Autodesk Inventor part; units mm, degrees
ref_plane "YZ Plane" through (0, 0, 0) normal (1, 0, 0) x (0, 1, 0)
ref_plane "XZ Plane" through (0, 0, 0) normal (0, 1, 0) x (-1, 0, 0)
ref_plane "XY Plane" through (0, 0, 0) normal (0, 0, 1) x (1, 0, 0)
sketch "Sketch1" plane through (0, 0, 0) normal (0, 0, 1) x (1, 0, 0)
  line L0 (0, 0) -> (177.8, 0)
  line L1 (177.8, 0) -> (177.8, 101.6)
  line L2 (177.8, 101.6) -> (0, 101.6)
  line L3 (0, 101.6) -> (0, 0)
  arc A0 (25.4, 101.6) -> (0, 76.2) centre (25.4, 76.2) ccw
  arc A1 (177.8, 76.2) -> (152.4, 101.6) centre (152.4, 76.2) ccw
  arc A2 (152.4, 0) -> (177.8, 25.4) centre (152.4, 25.4) ccw
  arc A3 (0, 25.4) -> (25.4, 0) centre (25.4, 25.4) ccw
  arc A4 (88.9, 85.09) -> (54.61, 50.8) centre (88.9, 50.8) ccw construction
  arc A5 (88.9, 88.9) -> (50.8, 50.8) centre (88.9, 50.8) ccw
  arc A6 (88.9, 81.28) -> (58.42, 50.8) centre (88.9, 50.8) ccw
  arc A7 (88.9, 81.28) -> (88.9, 88.9) centre (88.9, 85.09) ccw
  arc A8 (50.8, 50.8) -> (58.42, 50.8) centre (54.61, 50.8) ccw
  line L4 (88.9, 50.8) -> (54.61, 50.8) construction
  line L5 (88.9, 50.8) -> (88.9, 85.09) construction
  arc A9 (88.9, 20.32) -> (119.38, 50.8) centre (88.9, 50.8) ccw
  line L6 (88.9, 50.8) -> (123.19, 50.8) construction
  arc A10 (88.9, 16.51) -> (123.19, 50.8) centre (88.9, 50.8) ccw construction
  arc A11 (127, 50.8) -> (119.38, 50.8) centre (123.19, 50.8) ccw
  arc A12 (88.9, 12.7) -> (127, 50.8) centre (88.9, 50.8) ccw
  arc A13 (88.9, 20.32) -> (88.9, 12.7) centre (88.9, 16.51) ccw
  line L7 (0, 50.8) -> (177.8, 50.8)
  line L8 (88.9, 101.6) -> (88.9, 0)
  circle A14 centre (12.7, 71.882) radius 6.35
  circle A15 centre (33.02, 71.882) radius 6.35
  circle A16 centre (12.7, 29.718) radius 6.35
  circle A17 centre (33.02, 29.718) radius 6.35
  circle A18 centre (165.1, 29.718) radius 6.35
  circle A19 centre (144.78, 29.718) radius 6.35
  circle A20 centre (165.1, 71.882) radius 6.35
  circle A21 centre (144.78, 71.882) radius 6.35
  point P0 (0, 0)
  point P1 (0, 0)
  point P2 (-19.4884, -65.4138)
  dimension "d2" = 177.8
  dimension "d3" = 101.6
  dimension "d4" = 50.8
  dimension "d5" = 50.8
  dimension "d6" = 50.8
  dimension "d7" = 50.8
  dimension "d9" = 50.8
  dimension "d10" = 88.9
  dimension "d11" = 34.29
  dimension "d12" = 90
  dimension "d13" = 7.62
  dimension "d14" = 360
  dimension "d15" = 0
  dimension "d16" = 0
  dimension "d17" = 0
  dimension "d19" = 0
  dimension "d20" = 12.7
  dimension "d21" = 12.7
  dimension "d22" = 20.32
  dimension "d24" = 21.082
  dimension "d25" = 12.7
extrude "Extrusion1" add sketch "Sketch1" along normal blind 3.175 contours A3 L3 L7 A8 L8 A13 L0 | L8 A12 L7 L1 A2 L0 | L3 A0 L2 L8 A5 L7 | A11 L7 L8 A7 L2 A1 L1 | L8 L7 A9 | A6 L8 L7
sketch "Sketch2" plane through (0, 0, 3.175) normal (0, 0, 1) x (1, 0, 0)
  line L0 (0, 0) -> (177.8, 0)
  line L1 (177.8, 0) -> (177.8, 101.6)
  line L2 (177.8, 101.6) -> (0, 101.6)
  line L3 (0, 101.6) -> (0, 0)
  circle A0 centre (12.7, 71.882) radius 6.35
  circle A1 centre (12.7, 71.882) radius 6.35
  circle A2 centre (33.02, 71.882) radius 6.35
  circle A3 centre (12.7, 29.718) radius 6.35
  circle A4 centre (33.02, 29.718) radius 6.35
  circle A5 centre (33.02, 71.882) radius 6.35
  circle A6 centre (12.7, 29.718) radius 6.35
  circle A7 centre (33.02, 29.718) radius 6.35
  circle A8 centre (144.78, 71.882) radius 6.35
  circle A9 centre (144.78, 29.718) radius 6.35
  circle A10 centre (165.1, 71.882) radius 6.35
  circle A11 centre (165.1, 29.718) radius 6.35
  circle A12 centre (144.78, 71.882) radius 6.35
  circle A13 centre (165.1, 71.882) radius 6.35
  circle A14 centre (144.78, 29.718) radius 6.35
  circle A15 centre (165.1, 29.718) radius 6.35
  arc A16 (88.9, 85.09) -> (54.61, 50.8) centre (88.9, 50.8) ccw construction
  arc A17 (88.9, 93.98) -> (45.72, 50.8) centre (88.9, 50.8) ccw
  arc A18 (88.9, 76.2) -> (63.5, 50.8) centre (88.9, 50.8) ccw
  arc A19 (88.9, 76.2) -> (88.9, 93.98) centre (88.9, 85.09) ccw
  arc A20 (45.72, 50.8) -> (63.5, 50.8) centre (54.61, 50.8) ccw
  line L4 (88.9, 50.8) -> (54.61, 50.8) construction
  line L5 (88.9, 50.8) -> (88.9, 85.09) construction
  arc A21 (88.9, 25.4) -> (114.3, 50.8) centre (88.9, 50.8) ccw
  line L6 (88.9, 50.8) -> (123.19, 50.8) construction
  arc A22 (88.9, 16.51) -> (123.19, 50.8) centre (88.9, 50.8) ccw construction
  arc A23 (88.9, 7.62) -> (132.08, 50.8) centre (88.9, 50.8) ccw
  arc A24 (132.08, 50.8) -> (114.3, 50.8) centre (123.19, 50.8) ccw
  arc A25 (88.9, 25.4) -> (88.9, 7.62) centre (88.9, 16.51) ccw
  arc A26 (25.4, 101.6) -> (0, 76.2) centre (25.4, 76.2) ccw
  arc A27 (0, 25.4) -> (25.4, 0) centre (25.4, 25.4) ccw
  line L7 (177.8, 25.4) -> (177.8, 76.2)
  arc A28 (152.4, 0) -> (177.8, 25.4) centre (152.4, 25.4) ccw
  arc A29 (129.8378, 37.0665) -> (128.016, 32.512) centre (152.4, 25.4) ccw
  arc A30 (177.8, 76.2) -> (152.4, 101.6) centre (152.4, 76.2) ccw
  arc A31 (177.8, 76.2) -> (152.4, 101.6) centre (152.4, 76.2) ccw
  dimension "d28" = 177.8
  dimension "d29" = 101.6
  dimension "d30" = 12.7
  dimension "d31" = 12.7
  dimension "d32" = 12.7
  dimension "d33" = 12.7
  dimension "d34" = 12.7
  dimension "d35" = 12.7
  dimension "d36" = 12.7
  dimension "d37" = 12.7
  dimension "d38" = 34.29
  dimension "d39" = 90
  dimension "d40" = 17.78
  dimension "d41" = 50.8
  dimension "d42" = 88.9
  dimension "d45" = 360
  dimension "d48" = 25.4
  dimension "d49" = 50.8
  dimension "d57" = 50.8
extrude "Extrusion2" add sketch "Sketch2" along normal blind 3.175 contours A27 L3 A26 L2 A30 L1 A28 L0
sketch "Sketch3" plane through (177.8, 25.4, 0) normal (1, 0, 0) x (0, 0, -1)
  line L0 (-6.35, 0) -> (-6.35, 50.8)
  line L1 (-6.35, 50.8) -> (0, 50.8)
  line L2 (0, 50.8) -> (0, -25.4)
  line L3 (0, -25.4) -> (-6.35, -25.4)
  line L4 (-6.35, -25.4) -> (-6.35, 50.8)
extrude "Extrusion3" cut sketch "Sketch3" against normal blind 3.048
sketch "Sketch4" plane through (0, 25.4, 0) normal (-1, 0, 0) x (0, 0, 1)
  line L0 (6.35, 50.8) -> (0, 50.8)
  line L1 (6.35, -25.4) -> (6.35, 0)
  line L2 (0, 50.8) -> (6.35, 50.8)
  line L3 (6.35, 50.8) -> (6.35, -25.4)
  line L4 (6.35, -25.4) -> (0, -25.4)
  line L5 (0, -25.4) -> (0, 50.8)
  point P0 (0, -25.4)
extrude "Extrusion4" cut sketch "Sketch4" against normal blind 3.048
sketch "Sketch5" plane through (25.4, 0, 0) normal (0, -1, 0) x (1, 0, 0)
  line L0 (-22.352, 6.35) -> (-22.352, 0)
  line L1 (149.352, 6.35) -> (149.352, 0)
  line L2 (-22.352, 6.35) -> (149.352, 6.35)
  line L3 (149.352, 6.35) -> (149.352, 0)
  line L4 (149.352, 0) -> (-22.352, 0)
  line L5 (-22.352, 0) -> (-22.352, 6.35)
  point P0 (-25.4, 0)
extrude "Extrusion5" cut sketch "Sketch5" against normal blind 3.048
sketch "Sketch6" plane through (0, 0, 6.35) normal (0, 0, 1) x (1, 0, 0)
  arc A0 (3.048, 28.448) -> (28.448, 3.048) centre (28.448, 28.448) ccw
  arc A1 (149.352, 3.048) -> (174.752, 28.448) centre (149.352, 28.448) ccw
  line L0 (3.048, 76.2) -> (3.048, 13.3357)
  line L1 (13.3357, 3.048) -> (164.4643, 3.048)
  line L2 (174.752, 13.3357) -> (174.752, 76.2)
  line L3 (3.048, 28.448) -> (3.048, 3.048)
  line L4 (3.048, 3.048) -> (28.448, 3.048)
  line L5 (174.752, 28.448) -> (174.752, 3.048)
  line L6 (149.352, 3.048) -> (174.752, 3.048)
  point P0 (0, 0)
  point P1 (3.048, 13.3357)
  dimension "d66" = 50.8
  dimension "d67" = 50.8
extrude "Extrusion6" cut sketch "Sketch6" against normal through all
properties part number "Back_plate"
The model under review builds one solid part; all positions refer to its coordinate system, in mm. A direction names the side the tool comes from. Round coordinates to 2 decimals unless told otherwise and drop trailing zeros. Order: outer loops, then holes, each group sorted by start corner. A loop starts at its lowest first (then second) coordinate and runs counter-clockwise, first axis right, second up. Notation, with made-up numbers: (20, 80.5) -> (66, 80.5) arc R17 cw to (66, 100.5) -> close; hole circle Ø9 at (5, 19). An arc over 180 degrees is marked (long way). One line per item, written item: value. Start each with the question number.
Q1. Take a section at B-B (y = 85.09). Write out the cut boundary in (x, z) (3 decimals), and give its area (3 significant figures).
Q2. Take a section at D-D (x = 54.61). Write out the cut boundary in (y, z) (3 decimals).
Q3. Mouldability with a two-part tool opening along Y and no side actions: class faces 1 (the face through (8.02, 25.426, 3.131)), 2 (the face through (7.24, 93.96, 3.13)), 3 (the face through (88, 3.048, 3)) as released by +Y, released by -Y, zero draft, split by the parting line, or undercut.
Q4. Machinability: for faces 4 (the face through (68, 72, 3.175)), 5 (the face through (61.66, 77.44, 1.57)), 6 (the face through (170.16, 94.36, 3.13)), which of the approach directions +Z, -Z, +X, -X, +Y, -Y give a long, thin tool a straight path to every point of the face, cutting with its end or side? Answer none if there is none.
Q5. Take a section at A-A (x = 144.78). Write out the cut boundary in (y, z), and give its area (3 significant figures).
Q6. Wall thickness on line 1 (Y direction, x = 144.78, z = 5.25); line 2 (Y direction, x = 12.7, z = 3.25); line 3 (X direction, y = 31.5, z = 4.75): over which ranges is each line inside the solid? List them lowest first.
Q7. Clearance check with flat-ended pins moving along their axes: pin 1 Ø1.9 at (y, z) = (48, 2.5) entering from +X; pin 2 Ø2 at (y, z) = (85.5, 4) entering from +X; pin 3 Ø16.5 at (x, y) = (33.02, 29.718) entering from -Z; pin 4 Ø7.5 at (x, y) = (165.1, 29.718) entering from -Z. State where each tip first meets the part, or that it passes through.
Q8. Take a section at C-C (z = 1). Count the separate pieces of the cut face and the enclosed holes in it, and give its area (3 significant figures).
Reported:
1. outline: (1.607, 0) -> (72.293, 0) -> (72.293, 3.175) -> (62.657, 3.175) -> (62.657, 6.35) -> (1.607, 6.35) -> close; (92.71, 0) -> (176.193, 0) -> (176.193, 6.35) -> (97.79, 6.35) -> (97.79, 3.175) -> (92.71, 3.175) -> close
1. area: 932 mm2
2. outline: (3.048, 0) -> (46.99, 0) -> (46.99, 3.175) -> (41.91, 3.175) -> (41.91, 6.35) -> (3.048, 6.35) -> close; (67.407, 0) -> (101.6, 0) -> (101.6, 6.35) -> (77.043, 6.35) -> (77.043, 3.175) -> (67.407, 3.175) -> close
3. face 1: undercut
3. face 2: released by +Y
3. face 3: released by -Y
4. face 4: +Z
4. face 5: +Z, -Z
4. face 6: +Z, -Z, +X, +Y
5. outline: (3.05, 0) -> (23.37, 0) -> (23.37, 6.35) -> (3.05, 6.35) -> close; (36.07, 0) -> (65.53, 0) -> (65.53, 6.35) -> (36.07, 6.35) -> close; (78.23, 0) -> (101.6, 0) -> (101.6, 6.35) -> (78.23, 6.35) -> close
5. area: 465 mm2
6. line 1: y = 3.05 to 23.37, 36.07 to 65.53, 78.23 to 101.6
6. line 2: y = 8.52 to 23.37, 36.07 to 65.53, 78.23 to 98.2
6. line 3: x = 3.05 to 6.61, 18.79 to 26.93, 39.11 to 105.41, 127.53 to 138.69, 150.87 to 159.01, 171.19 to 174.75
7. pin 1: stops at x = 174.75
7. pin 2: stops at x = 176.41
7. pin 3: stops at z = 0
7. pin 4: passes through
8. separate pieces: 1
8. enclosed holes: 10
8. area: 14,600 mm2
